from build123d import *

# Parameters (mm, degrees)
F1_R      = 4.25
F2_DEPTH  = 3
F4_DEPTH  = 10
F8_DEPTH  = 3.001
F10_DEPTH = 8.5
F11_R     = 1.55
F12_DEPTH = 91.501
F13_R     = 1.55
F14_DEPTH = 91.501
F15_R     = 1.55
F16_DEPTH = 96.951
F17_R     = 1.55
F18_DEPTH = 96.951
F20_DEPTH = 10


with BuildPart() as f2:
    # F1 (on Top) → F2 (new body)
    with BuildSketch(Plane.XY):
        Polygon((41.5, 41.5), (41.5, 50), (-41.5, 50), (-41.5, 41.5), (-50, 41.5), (-50, -41.5), (-41.5, -41.5), (-41.5, -50), (41.5, -50), (41.5, -41.5), (50, -41.5), (50, 41.5), align=None)
        Circle(F1_R, mode=Mode.SUBTRACT)
    extrude(amount=F2_DEPTH)

    # F3 (on face) → F4 (join)
    with BuildSketch(Plane.XY.offset(3)):
        Polygon((31.05, 43.95), (39.55, 43.95), (39.55, 39.55), (43.95, 39.55), (43.95, 31.05), (46.95, 31.05), (46.95, 39.55), (50, 39.55), (50, 41.5), (41.5, 41.5), (41.5, 50), (39.55, 50), (39.55, 46.95), (31.05, 46.95), align=None)
    extrude(amount=F4_DEPTH)

    # F5: F2 across plane


with BuildPart() as f2_1:
    add(f2.part)
    add(f2.part.mirror(Plane.YZ))

    # F6: F2 across plane


with BuildPart() as f2_2:
    add(f2_1.part)
    add(f2_1.part.mirror(Plane.XZ))

    # F7 (on face) → F8 (cut, through all)
    with BuildSketch(Plane.XY.offset(3)):
        with BuildLine():
            ThreePointArc((-36.5857864376, 32.3431457505), (-38.7653668647, 32.7766912532), (-40, 30.9289321881))
            Line((-40, 30.9289321881), (-40, -30.9289321881))
            ThreePointArc((-40, -30.9289321881), (-38.7653668647, -32.7766912532), (-36.5857864376, -32.3431457505))
            Line((-36.5857864376, -32.3431457505), (-8.8666891252, -4.6240484381))
            ThreePointArc((-8.8666891252, -4.6240484381), (-10, 0), (-8.8666891252, 4.6240484381))
            Line((-8.8666891252, 4.6240484381), (-36.5857864376, 32.3431457505))
        make_face()
        with BuildLine():
            Line((30.9289321881, 40), (-30.9289321881, 40))
            ThreePointArc((-30.9289321881, 40), (-32.7766912532, 38.7653668647), (-32.3431457505, 36.5857864376))
            Line((-32.3431457505, 36.5857864376), (-4.6240484381, 8.8666891252))
            ThreePointArc((-4.6240484381, 8.8666891252), (0, 10), (4.6240484381, 8.8666891252))
            Line((4.6240484381, 8.8666891252), (32.3431457505, 36.5857864376))
            ThreePointArc((32.3431457505, 36.5857864376), (32.7766912532, 38.7653668647), (30.9289321881, 40))
        make_face()
        with BuildLine():
            Line((40, -30.9289321881), (40, 30.9289321881))
            ThreePointArc((40, 30.9289321881), (38.7653668647, 32.7766912532), (36.5857864376, 32.3431457505))
            Line((36.5857864376, 32.3431457505), (8.8666891252, 4.6240484381))
            ThreePointArc((8.8666891252, 4.6240484381), (10, 0), (8.8666891252, -4.6240484381))
            Line((8.8666891252, -4.6240484381), (36.5857864376, -32.3431457505))
            ThreePointArc((36.5857864376, -32.3431457505), (38.7653668647, -32.7766912532), (40, -30.9289321881))
        make_face()
        with BuildLine():
            ThreePointArc((-32.3431457505, -36.5857864376), (-32.7766912532, -38.7653668647), (-30.9289321881, -40))
            Line((-30.9289321881, -40), (30.9289321881, -40))
            ThreePointArc((30.9289321881, -40), (32.7766912532, -38.7653668647), (32.3431457505, -36.5857864376))
            Line((32.3431457505, -36.5857864376), (4.6240484381, -8.8666891252))
            ThreePointArc((4.6240484381, -8.8666891252), (0, -10), (-4.6240484381, -8.8666891252))
            Line((-4.6240484381, -8.8666891252), (-32.3431457505, -36.5857864376))
        make_face()
    extrude(amount=-F8_DEPTH, mode=Mode.SUBTRACT)

    # F9 (on face) → F10 (join)
    with BuildSketch(Plane.XY.offset(13)):
        Polygon((41.5, 50), (39.55, 50), (39.55, 39.55), (50, 39.55), (50, 41.5), (41.5, 41.5), align=None)
        Polygon((-41.5, 41.5), (-50, 41.5), (-50, 39.55), (-39.55, 39.55), (-39.55, 50), (-41.5, 50), align=None)
        Polygon((39.55, -39.55), (39.55, -50), (41.5, -50), (41.5, -41.5), (50, -41.5), (50, -39.55), align=None)
        Polygon((-41.5, -50), (-39.55, -50), (-39.55, -39.55), (-50, -39.55), (-50, -41.5), (-41.5, -41.5), align=None)
    extrude(amount=F10_DEPTH)

    # F11 (on face) → F12 (cut, through all)
    with BuildSketch(Plane(origin=(-41.5, 0, 0), x_dir=(0, -1, 0), z_dir=(-1, 0, 0))):
        with Locations((45.75, 17.25)):
            Circle(F11_R)
        with Locations((-45.75, 17.25)):
            Circle(F11_R)
    extrude(amount=-F12_DEPTH, mode=Mode.SUBTRACT)

    # F13 (on face) → F14 (cut, through all)
    with BuildSketch(Plane(origin=(0, 41.5, 0), x_dir=(-1, 0, 0), z_dir=(0, 1, 0))):
        with Locations((45.75, 17.25)):
            Circle(F13_R)
        with Locations((-45.75, 17.25)):
            Circle(F13_R)
    extrude(amount=-F14_DEPTH, mode=Mode.SUBTRACT)

    # F15 (on face) → F16 (cut, through all)
    with BuildSketch(Plane(origin=(-46.95, 0, 0), x_dir=(0, -1, 0), z_dir=(-1, 0, 0))):
        with Locations((-35.3, 8)):
            Circle(F15_R)
        with Locations((35.3, 8)):
            Circle(F15_R)
    extrude(amount=-F16_DEPTH, mode=Mode.SUBTRACT)

    # F17 (on face) → F18 (cut, through all)
    with BuildSketch(Plane(origin=(0, 46.95, 0), x_dir=(-1, 0, 0), z_dir=(0, 1, 0))):
        with Locations((-35.3, 8)):
            Circle(F17_R)
        with Locations((35.3, 8)):
            Circle(F17_R)
    extrude(amount=-F18_DEPTH, mode=Mode.SUBTRACT)

    # F19 (on face) → F20 (join)
    with BuildSketch(Plane.XY.offset(3)):
        Polygon((21.0073593129, 25.25), (25.25, 25.25), (25.25, 21.0073593129), (28.7855339059, 24.5428932188), (24.5428932188, 28.7855339059), align=None)
        Polygon((-25.25, 21.0073593129), (-25.25, 25.25), (-21.0073593129, 25.25), (-24.5428932188, 28.7855339059), (-28.7855339059, 24.5428932188), align=None)
        Polygon((-21.0073593129, -25.25), (-25.25, -25.25), (-25.25, -21.0073593129), (-28.7855339059, -24.5428932188), (-24.5428932188, -28.7855339059), align=None)
        Polygon((25.25, -21.0073593129), (25.25, -25.25), (21.0073593129, -25.25), (24.5428932188, -28.7855339059), (28.7855339059, -24.5428932188), align=None)
    extrude(amount=F20_DEPTH)


solid = f2_2.part
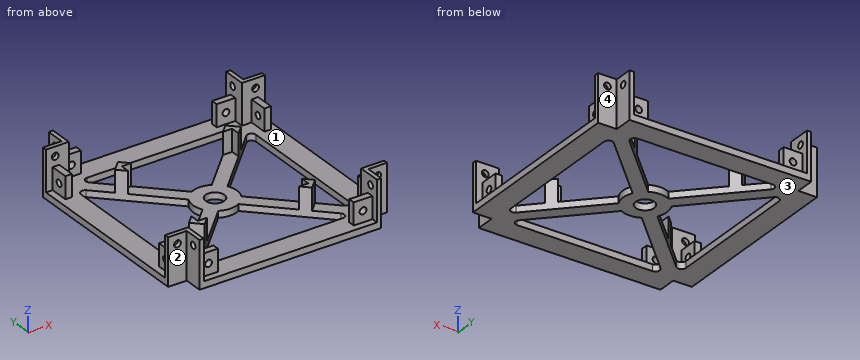
Verification items for the finished model (mm, model axes). Face numbers are marked on the shaded views. Give positions to 0.01 mm unless a question says otherwise; leave off trailing zeros. Loops run counter-clockwise (first coordinate to the right, second up) from the corner with the lowest first, then second, coordinate; pieces in that order, holes last.
1) Thickness scan on line 1 along X through (y, z) = (0, 2); line 2 along X through (y, z) = (-32, 9); line 3 along Z through (x, y) = (41.15, -45.75). Record the ranges inside material, lowest first.
2) Draft check along Y on the marked faces 1, 2, 3 and 4. Enter one of: pulls with the +Y half, pulls with the -Y half, needs draft (parallel to the pull), parting line crosses it, or undercut.
3) Sectioned sample at D-D, the plane y = 19. Enter the section's corners in (x, z).
4) Sectioned sample at C-C, the plane z = 4.25. Count the separate pieces of the cut face and the enclosed holes in it, then the cut area to 3 significant figures.
5) Sectioned sample at A-A, the plane x = 45.75. Enter the section's corners in (y, z).
6) Depth check by flat-ended pin: pin 1 Ø3.5 at (y, z) = (-45.5, 8.5) entering from +X; pin 2 Ø10 at (x, y) = (31.5, 20.5) entering from -Z; pin 3 Ø1.5 at (y, z) = (-45.5, 10) entering from -X; pin 4 Ø5 at (y, z) = (29.5, 6.5) entering from +X. Enter the tip coordinate at first touch or a pass-through.
Answers:
1. line 1: x = -50 to -40, -10 to -4.25, 4.25 to 10, 40 to 50
1. line 2: x = -46.95 to -43.95, 43.95 to 46.95
1. line 3: z = 0 to 15.7, 18.8 to 21.5
2. face 1: undercut
2. face 2: pulls with the -Y half
2. face 3: needs draft
2. face 4: pulls with the +Y half
3. outline: (-50, 0) - (-40, 0) - (-40, 3) - (-50, 3) - close; (-23.24, 0) - (-14.76, 0) - (-14.76, 3) - (-23.24, 3) - close; (14.76, 0) - (23.24, 0) - (23.24, 3) - (14.76, 3) - close; (40, 0) - (50, 0) - (50, 3) - (40, 3) - close
4. separate pieces: 8
4. enclosed holes: 0
4. area: 436 mm2
5. outline: (-41.5, 0) - (41.5, 0) - (41.5, 15.7) - (39.55, 15.7) - (39.55, 13) - (31.05, 13) - (31.05, 3) - (-31.05, 3) - (-31.05, 13) - (-39.55, 13) - (-39.55, 15.7) - (-41.5, 15.7) - close; (-41.5, 18.8) - (-39.55, 18.8) - (-39.55, 21.5) - (-41.5, 21.5) - close; (39.55, 18.8) - (41.5, 18.8) - (41.5, 21.5) - (39.55, 21.5) - close; hole circle Ø3.1 at (-35.3, 8); hole circle Ø3.1 at (35.3, 8)
6. pin 1: stops at x = 41.5
6. pin 2: stops at z = 0
6. pin 3: stops at x = -41.5
6. pin 4: stops at x = 46.95
